The figure shows three views and two pictorial views of one solid part (mm, origin at its lowest corner). Answer the questions. Coordinates: 2 decimals unless noted, no trailing zeros. Order: outer loops, then holes, each group sorted by start corner. A loop starts at its lowest first (then second) coordinate and runs counter-clockwise, first axis right, second up. Notation, with made-up numbers: (35.25, 50) -> (66.25, 50) arc R26 cw to (66.25, 85) -> close; hole circle Ø2 at (55, 67). An arc over 180 degrees is marked (long way). Return JSON: item names as keys, results as strings.
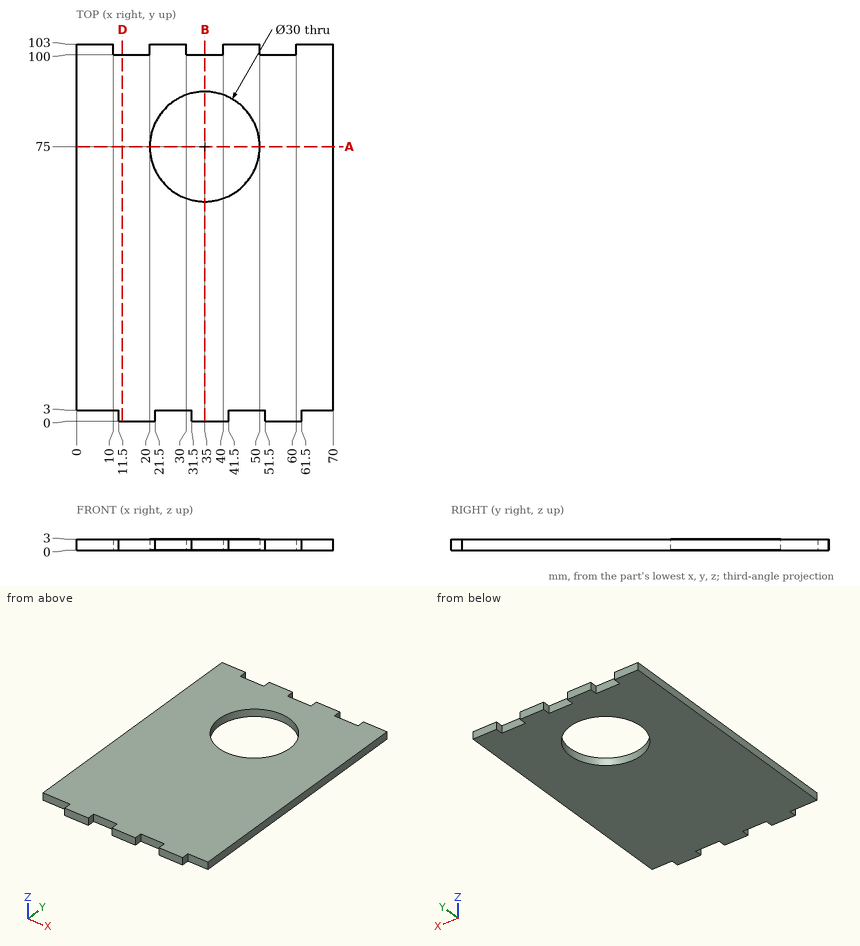
1. Each of these flat-tipped pins is pushed along its axis until it touches: pin 1 Ø1.5 at (y, z) = (2, 1) entering from +X; pin 2 Ø1.5 at (x, z) = (5, 2) entering from -Y; pin 3 Ø0.9 at (y, z) = (2, 1) entering from -X. Where does it stop, or does it pass through?
Answer block:
{"pin 1": "stops at x = 61.5", "pin 2": "stops at y = 3", "pin 3": "stops at x = 11.5"}
2. The part is cut by section D-D on x = 12.5. Give the vertices of the cut face in (y, z), and give its area (3 significant figures).
Answer block:
{"outline": "(0, 0) -> (100, 0) -> (100, 3) -> (0, 3) -> close", "area": "300 mm2"}
3. Consider line 1 (Y direction, x = 35, z = 1.15); line 2 (Y direction, x = 54, z = 0.75); line 3 (X direction, y = 80, z = 2.55). Determine where each line is inside the solid, lowest interval first. Write a range as from..to.
Answer block:
{"line 1": "y = 0..60, 90..100", "line 2": "y = 0..100", "line 3": "x = 0..20.86, 49.14..70"}
4. The part is cut by section B-B on x = 35. Give the vertices of the cut face in (y, z).
Answer block:
{"outline": "(0, 0) -> (60, 0) -> (60, 3) -> (0, 3) -> close; (90, 0) -> (100, 0) -> (100, 3) -> (90, 3) -> close"}
5. The part is cut by section A-A on y = 75. Give the vertices of the cut face in (x, z).
Answer block:
{"outline": "(0, 0) -> (20, 0) -> (20, 3) -> (0, 3) -> close; (50, 0) -> (70, 0) -> (70, 3) -> (50, 3) -> close"}
